Autodesk Inventor part; units mm, degrees
ref_plane "YZ Plane" through (0, 0, 0) normal (1, 0, 0) x (0, 1, 0)
ref_plane "XZ Plane" through (0, 0, 0) normal (0, 1, 0) x (-1, 0, 0)
ref_plane "XY Plane" through (0, 0, 0) normal (0, 0, 1) x (1, 0, 0)
sketch "Sketch1" plane through (0, 0, 0) normal (0, 0, 1) x (1, 0, 0)
  line L0 (0, 0) -> (0, 50.8)
  line L1 (-12.3149, 50.587) -> (-12.3149, 50.587)
  arc A0 (76.2, 50.8) -> (0, 50.8) centre (38.1, 50.8) ccw
  line L2 (0, 0) -> (15.875, 0)
  line L3 (15.875, 0) -> (15.875, 50.8)
  arc A1 (60.325, 50.8) -> (15.875, 50.8) centre (38.1, 50.8) ccw
  line L4 (76.2, 50.8) -> (60.325, 50.8)
  line L5 (8.5732, 88.9) -> (68.624, 88.9) construction
  dimension "d1" = 15.875
  dimension "d3" = 50.8
  dimension "d6" = 38.1
extrude "Extrusion1" add sketch "Sketch1" along normal blind 15.875
equation "\"d4\" = d1"
properties part number "TelescopeHook"
Work out the finished part from the listing and answer in its coordinate system (mm). Coordinates: 2 decimals unless noted, no trailing zeros. Write each loop counter-clockwise with the first axis right and the second up, starting at its lowest first coordinate (ties: lowest second). Pieces come first, ordered by that corner, then holes. Notation, with made-up numbers: M 36.5,9 L 72.5,9 A19 cw 72.5,46 Z; hole C 77,-17 d5. An arc over 180 degrees is marked long. Answer as CSV lines item,"result". Start each with the question number.
Item 1: Section C-C on y = 33.5 is taken. Write down the section's boundary in (x, z) (3 decimals).
Item 2: Section A-A on y = 54.5 is taken. Write down the section's boundary in (x, z) (3 decimals).
Item 3: Consider L1, parallel to X at y = 51.5, z = 4.25; L2, parallel to X at y = 23, z = 5.75 (3 decimals); L3, parallel to X at y = 69.5, z = 5.25. Determine where each line is inside the solid, lowest interval first.
Item 4: Determine the mould class of faces 1 (the face through (37.26, 88.89, 7.83)), 2 (the face through (15.875, 25, 8)), 3 (the face through (68, 50.8, 8)), 4 (the face through (37.61, 73.02, 7.83)) for opening direction X: released by +X, released by -X, zero draft, split by the parting line, or undercut.
Item 5: Flat-ended cylindrical pins translate along their axes: P1, Ø3, axis at x = 24, z = 9.5, coming from the +Y side; P2, Ø8, axis at x = 65, z = 5, coming from the -Y side; P3, Ø6, axis at x = 32, z = 10, coming from the -Y side; P4, Ø6, axis at x = 24.5, y = 60.5, coming from the +Z side. Find the tip coordinate at first contact, or state that the pin passes through.
Item 6: Section D-D on x = 38.1 is taken. Write down the section's boundary in (y, z) (3 decimals), and give its area (3 significant figures).
Item 7: Section B-B on z = 3 is taken. Write down the section's boundary in (x, y) (3 decimals).
Checks:
1,outline,"M 0,0 L 15.875,0 L 15.875,15.875 L 0,15.875 Z"
2,outline,"M 0.18,0 L 16.185,0 L 16.185,15.875 L 0.18,15.875 Z; M 60.015,0 L 76.02,0 L 76.02,15.875 L 60.015,15.875 Z"
3,L1,"x = 0.01 to 15.89, 60.31 to 76.19"
3,L2,"x = 0 to 15.875"
3,L3,"x = 4.9 to 26.09, 50.11 to 71.3"
4,face 1,"split by the parting line"
4,face 2,"released by +X"
4,face 3,"zero draft"
4,face 4,"undercut"
5,P1,"stops at y = 86.76"
5,P2,"stops at y = 50.8"
5,P3,"stops at y = 71.08"
5,P4,"passes through"
6,outline,"M 73.025,0 L 88.9,0 L 88.9,15.875 L 73.025,15.875 Z"
6,area,"252 mm²"
7,outline,"M 0,0 L 15.875,0 L 15.875,50.8 A22.225 cw 60.325,50.8 L 76.2,50.8 A38.1 ccw 0,50.8 Z"
